```python
from build123d import *

# Parameters (mm, degrees)
BOSS_EXTRUDE1_DEPTH = 15
CUT_EXTRUDE1_DEPTH  = 10.5
CHAMFER1_SIZE       = 10


with BuildPart() as part:
    # Sketch1 → Boss-Extrude1 (new body)
    with BuildSketch(Plane(origin=(0, 0, 0), x_dir=(1, 0, 0), z_dir=(0, 1, 0))):
        with BuildLine():
            Line((-197.5, 207.5), (197.5, 207.5))
            ThreePointArc((197.5, 207.5), (204.571067812, 204.571067812), (207.5, 197.5))
            Line((207.5, 197.5), (207.5, -197.5))
            ThreePointArc((207.5, -197.5), (204.571067812, -204.571067812), (197.5, -207.5))
            Line((197.5, -207.5), (-197.5, -207.5))
            ThreePointArc((-197.5, -207.5), (-204.571067812, -204.571067812), (-207.5, -197.5))
            Line((-207.5, -197.5), (-207.5, 197.5))
            ThreePointArc((-207.5, 197.5), (-204.571067812, 204.571067812), (-197.5, 207.5))
        make_face()
    extrude(amount=-BOSS_EXTRUDE1_DEPTH)

    # Sketch2 → Cut-Extrude1 (cut)
    with BuildSketch(Plane.XZ.offset(15)):
        Polygon((-190, -200), (190, -200), (200, -190), (200, 190), (190, 200), (-190, 200), (-200, 190), (-200, -190), align=None)
        with BuildLine():
            Line((-175, -195), (175, -195))
            ThreePointArc((175, -195), (189.142135624, -189.142135624), (195, -175))
            Line((195, -175), (195, 175))
            ThreePointArc((195, 175), (189.142135624, 189.142135624), (175, 195))
            Line((175, 195), (-175, 195))
            ThreePointArc((-175, 195), (-189.142135624, 189.142135624), (-195, 175))
            Line((-195, 175), (-195, -175))
            ThreePointArc((-195, -175), (-189.142135624, -189.142135624), (-175, -195))
        make_face(mode=Mode.SUBTRACT)
    extrude(amount=-CUT_EXTRUDE1_DEPTH, mode=Mode.SUBTRACT)

    # Chamfer1
    chamfer1_edges = [part.edges().sort_by_distance(p)[0] for p in [
        (189.142135624, -15, -189.142135624),
        (0, -15, -195),
        (-189.142135624, -15, -189.142135624),
        (-195, -15, 0),
        (-189.142135624, -15, 189.142135624),
        (0, -15, 195),
        (189.142135624, -15, 189.142135624),
        (195, -15, 0),
    ]]
    chamfer(chamfer1_edges, length=CHAMFER1_SIZE)


solid = part.part
```
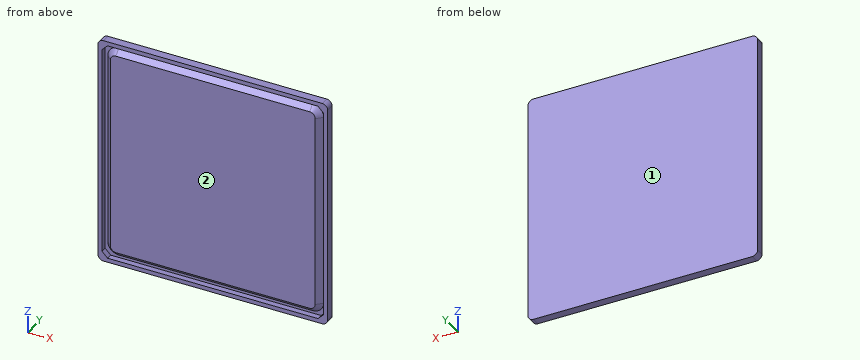
The listing builds one solid part. Answer for the finished solid, in the listing's coordinates (mm). Face numbers are marked on the shaded views. Give positions to 0.01 mm unless a question says otherwise; leave off trailing zeros. Write each loop counter-clockwise with the first axis right and the second up, starting at its lowest first coordinate (ties: lowest second). Pieces come first, ordered by that corner, then holes. Notation, with made-up numbers: (82, -19) - (90, -19) arc R20 cw to (90, -10) - close; hole circle Ø5 at (-29, 56). An arc over 180 degrees is marked (long way). Use one line per item in the form item = value. Start each with the question number.
1) Find section A-A on y = -10. Determine the outline of the cut face in (x, z).
2) Consider line 1 along X through (y, z) = (-5, -162); line 2 along X through (y, z) = (-9.5, -183); line 3 along Z through (x, y) = (162.5, -10.25). Determine where each line is inside the solid, lowest interval first. Write a range as from..to.
3) Find section C-C on x = -16. Determine the outline of the cut face in (y, z).
4) Find section B-B on z = -48. Determine the outline of the cut face in (x, y), plus the area to 3 significant figures.
5) The mould has two halves that part along Y. Classify the marked faces 1 and 2: pulls with the +Y half, pulls with the -Y half, needs draft (parallel to the pull), parting line crosses it, or undercut.
Geometry results:
q1.outline = (-207.5, -197.5) arc R10 ccw to (-197.5, -207.5) - (197.5, -207.5) arc R10 ccw to (207.5, -197.5) - (207.5, 197.5) arc R10 ccw to (197.5, 207.5) - (-197.5, 207.5) arc R10 ccw to (-207.5, 197.5) - close; (-190, -175) arc R15 ccw to (-175, -190) - (175, -190) arc R15 ccw to (190, -175) - (190, 175) arc R15 ccw to (175, 190) - (-175, 190) arc R15 ccw to (-190, 175) - close; hole (-200, -190) - (-190, -200) - (190, -200) - (200, -190) - (200, 190) - (190, 200) - (-190, 200) - (-200, 190) - close
q2.line_1 = -207.5..-200, -195..195, 200..207.5
q2.line_2 = -207.5..-200, -188.28..188.28, 200..207.5
q2.line_3 = -207.5..-200, -189.75..189.75, 200..207.5
q3.outline = (-15, -207.5) - (0, -207.5) - (0, 207.5) - (-15, 207.5) - (-15, 200) - (-4.5, 200) - (-4.5, 195) - (-5, 195) - (-15, 185) - (-15, -185) - (-5, -195) - (-4.5, -195) - (-4.5, -200) - (-15, -200) - close
q4.outline = (-207.5, -15) - (-200, -15) - (-200, -4.5) - (-195, -4.5) - (-195, -5) - (-185, -15) - (185, -15) - (195, -5) - (195, -4.5) - (200, -4.5) - (200, -15) - (207.5, -15) - (207.5, 0) - (-207.5, 0) - close
q4.area = 6,020 mm2
q5.face_1 = pulls with the +Y half
q5.face_2 = pulls with the -Y half
